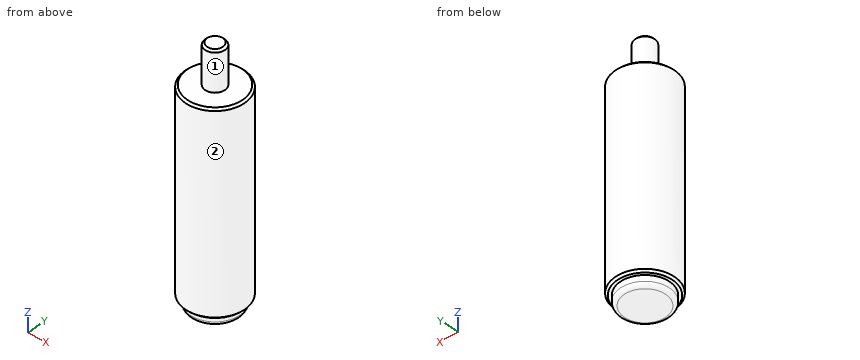
from build123d import *

# Parameters (mm, degrees)
F0_R     = 12.5
F1_DEPTH = 20
F3_R     = 15
F4_DEPTH = 100
F5_SIZE  = 1
F6_SIZE  = 1
F7_R     = 5
F8_DEPTH = 20
F9_SIZE  = 1
F10_R    = 2


with BuildPart() as f1:
    # F0 (on Top) → F1 (new body)
    with BuildSketch(Plane.XY):
        Circle(F0_R)
    extrude(amount=F1_DEPTH)

    # F3 (on offset) → F4 (join)
    with BuildSketch(Plane.XY.offset(5)):
        Circle(F3_R)
    extrude(amount=F4_DEPTH)

    # F5
    f5_edges = [f1.edges().sort_by_distance(p)[0] for p in [
        (-15, 0, 5),
    ]]
    chamfer(f5_edges, length=F5_SIZE)

    # F6
    f6_edges = [f1.edges().sort_by_distance(p)[0] for p in [
        (-15, 0, 105),
    ]]
    chamfer(f6_edges, length=F6_SIZE)

    # F7 (on face) → F8 (join)
    with BuildSketch(Plane.XY.offset(105)):
        Circle(F7_R)
    extrude(amount=F8_DEPTH)

    # F9
    f9_edges = [f1.edges().sort_by_distance(p)[0] for p in [
        (-5, 0, 125),
    ]]
    chamfer(f9_edges, length=F9_SIZE)

    # F10
    f10_edges = [f1.edges().sort_by_distance(p)[0] for p in [
        (-12.5, 0, 0),
    ]]
    fillet(f10_edges, radius=F10_R)


solid = f1.part
For this review, take the finished solid that the model builds, in its own axes (mm). Face numbers are marked on the shaded views. A direction names the side the tool comes from. Give positions to 0.01 mm unless a question says otherwise; leave off trailing zeros. Loops run counter-clockwise (first coordinate to the right, second up) from the corner with the lowest first, then second, coordinate; pieces in that order, holes last. Notation, with made-up numbers: M -20,49 L 30,49 A17 cw 30,60 Z; hole C 3.25,-0.5 d5. An arc over 180 degrees is marked long. Answer as a JSON object with one key per item and string values. Group by question number.
Q1. For probe 1 along Z at (x, y) = (12.5, 6); probe 2 along Z at (x, y) = (-3, -9); probe 3 along Y at (x, z) = (0.25, 119), list the stretches that pass through material, from the lowest coordinate up. Write a range as [from, to].
Q2. Add section A-A on y = 0. Give the boundary of the cut face in (x, z), and give its area (3 significant figures).
Q3. Add section C-C on z = 31.5. Give the boundary of the cut face in (x, y), and give its area (3 significant figures).
Q4. Tool access review of the marked faces 1 and 2: name each direction out of +Z, -Z, +X, -X, +Y, -Y from which nothing blocks a thin tool from reaching the whole face with its end or side.
Q5. Insertion check: P1, Ø2, axis at y = 5, z = 76.5, coming from the +X side; P2, Ø1.5, axis at y = 9.5, z = 30.5, coming from the +X side; P3, Ø2, axis at x = -5.5, y = 8, coming from the +Z side. Each pin has a flat end and moves straight along its axis. Give the tip position at first contact, or say it passes through.
Checked values:
{
 "1": {"probe 1": "[5, 105]", "probe 2": "[0, 105]", "probe 3": "[-4.99, 4.99]"},
 "2": {"outline": "M -15,6 L -14,5 L -12.5,5 L -12.5,2 A2 ccw -10.5,0 L 10.5,0 A2 ccw 12.5,2 L 12.5,5 L 14,5 L 15,6 L 15,104 L 14,105 L 5,105 L 5,124 L 4,125 L -4,125 L -5,124 L -5,105 L -14,105 L -15,104 Z", "area": "3,320 mm²"},
 "3": {"outline": "C 0,0 d30", "area": "707 mm²"},
 "4": {"face 1": "+Z", "face 2": "+Z, -Z"},
 "5": {"P1": "x = 14.46", "P2": "x = 12.18", "P3": "z = 105"}
}
